Can you work these out from the model? Positions are in its coordinate system, mm. A direction names the side the tool comes from. Give positions to 0.01 mm unless a question says otherwise; leave off trailing zeros. Loops run counter-clockwise (first coordinate to the right, second up) from the corner with the lowest first, then second, coordinate; pieces in that order, holes last.
Autodesk Fusion 360 part; units mm, degrees
sketch "Sketch1" plane through (0, 0, 0) normal (0, 1, 0) x (1, 0, 0)
  line L0 (-22.3654, 14.0021) -> (11.8346, 14.0021)
  line L1 (11.8346, 14.0021) -> (11.8346, -7.1979)
  line L2 (11.8346, -7.1979) -> (-22.3654, -7.1979)
  line L3 (-22.3654, -7.1979) -> (-22.3654, 14.0021)
  line L4 (-19.5354, 11.0221) -> (-16.9954, 11.0221)
  line L5 (-16.9954, 11.0221) -> (-16.9954, -4.2179)
  line L6 (-16.9954, -4.2179) -> (-19.5354, -4.2179)
  line L7 (-19.5354, -4.2179) -> (-19.5354, 11.0221)
  line L8 (6.4646, 8.4821) -> (9.0046, 8.4821)
  line L9 (9.0046, 8.4821) -> (9.0046, -1.6779)
  line L10 (9.0046, -1.6779) -> (6.4646, -1.6779)
  line L11 (6.4646, -1.6779) -> (6.4646, 8.4821)
  line L12 (11.8346, 3.4021) -> (-22.3654, 3.4021) construction
  line L13 (-16.2654, 14.0021) -> (5.7346, 14.0021)
  line L14 (5.7346, 14.0021) -> (5.7346, -7.1979)
  line L15 (5.7346, -7.1979) -> (-16.2654, -7.1979)
  line L16 (-16.2654, -7.1979) -> (-16.2654, 14.0021)
  line L17 (-18.2654, -4.2179) -> (-18.2654, 11.0221) construction
  line L18 (7.7346, -1.6779) -> (7.7346, 8.4821) construction
  circle A0 centre (7.7346, 11.0021) radius 1.5
  circle A1 centre (7.7346, -4.1979) radius 1.5
  line L19 (7.7346, -4.1979) -> (7.7346, 11.0021) construction
  point P0 (-16.9954, 3.4021)
  point P1 (-19.5354, 3.4021)
  point P2 (6.4646, 3.4021)
  point P3 (9.0046, 3.4021)
  dimension "d1" = 34.2
  dimension "d2" = 21.2
  dimension "d3" = 15.24
  dimension "d4" = 2.54
  dimension "d5" = 10.16
  dimension "d6" = 2.54
  dimension "d7" = 22
  dimension "d8" = 4.1
  dimension "d9" = 4.1
  dimension "d16" = 3
  dimension "d17" = 3
  dimension "d18" = 15.2
extrude "Extrude1" add sketch "Sketch1" against normal blind 1.7 contours L0 L2 L3 L16 | L0 L2 L13 L14 L15 L16 | L0 L1 L2 L14 | L4 L5 L6 L7 | L8 L9 L10 L11 | A0 | A1
extrude "Extrude2" add sketch "Sketch1" along normal blind 2.2 contours L0 L2 L13 L14 L15 L16
extrude "Extrude3" add sketch "Sketch1" along normal blind 4.5 contours L4 L5 L6 L7 | L8 L9 L10 L11
extrude "Extrude4" cut sketch "Sketch1" against normal blind 5 contours A0 | A1
(1) Suppose I cut it at A-A on y = 1.25. List the corners of the cut face in (x, z) for me.
Returned:
outline: (-19.54, -11.02) - (-17, -11.02) - (-17, 4.22) - (-19.54, 4.22) - close; (-16.27, -14) - (5.73, -14) - (5.73, 7.2) - (-16.27, 7.2) - close; (6.46, -8.48) - (9, -8.48) - (9, 1.68) - (6.46, 1.68) - close
(2) Thinking about a two-plate mould opening in X: for faces 5 (the flat face through (-6, -1.7, -4)), 6 (the flat face through (5.735, 1, -4)), 7 (the flat face through (-22.365, -1, -3)), which applies, pulls with the +X half, pulls with the -X half, needs draft (parallel to the pull), parting line crosses it, or undercut?
Returned:
face 5: needs draft
face 6: undercut
face 7: pulls with the -X half
(3) Suppose I cut it at C-C on z = 3.75. List the corners of the cut face in (x, y) for me.
Returned:
outline: (-22.37, -1.7) - (6.3, -1.7) - (6.3, 0) - (5.73, 0) - (5.73, 2.2) - (-16.27, 2.2) - (-16.27, 0) - (-17, 0) - (-17, 4.5) - (-19.54, 4.5) - (-19.54, 0) - (-22.37, 0) - close; (9.17, -1.7) - (11.83, -1.7) - (11.83, 0) - (9.17, 0) - close
(4) Suppose I cut it at D-D on y = -0.75. List the corners of the cut face in (x, z) for me.
Returned:
outline: (-22.37, -14) - (11.83, -14) - (11.83, 7.2) - (-22.37, 7.2) - close; hole circle Ø3 at (7.73, -11); hole circle Ø3 at (7.73, 4.2)
(5) Which directions (+Z, -Z, +X, -X, +Y, -Y) give clear straight access to the entire face, cutting with the end or side of a thin tool? Please do faces 1 (the flat face through (-19.535, 2, -3)), 2 (the flat face through (-18, 2, 4.218)), 3 (the flat face through (6.465, 2, -3)), 4 (the flat face through (8, 2, -8.482)).
Returned:
face 1: +Z, -Z, -X, +Y
face 2: +Z, -X, +Y
face 3: +Z, -Z, +Y
face 4: -Z, +X, +Y
(6) Suppose I cut it at B-B on z = -6. List the corners of the cut face in (x, y) for me.
Returned:
outline: (-22.37, -1.7) - (11.83, -1.7) - (11.83, 0) - (9, 0) - (9, 4.5) - (6.46, 4.5) - (6.46, 0) - (5.73, 0) - (5.73, 2.2) - (-16.27, 2.2) - (-16.27, 0) - (-17, 0) - (-17, 4.5) - (-19.54, 4.5) - (-19.54, 0) - (-22.37, 0) - close
(7) Please list where these lines run through material, in increasing order: probe 1 along X at (y, z) = (0.25, 1.25); probe 2 along X at (y, z) = (0.25, 2.25); probe 3 along Y at (x, z) = (3, -6).
Returned:
probe 1: x = -19.54 to -17, -16.27 to 5.73, 6.46 to 9
probe 2: x = -19.54 to -17, -16.27 to 5.73
probe 3: y = -1.7 to 2.2
(8) Will these pins go through, and if not, where does the flat tip stop? P1, Ø1.3, axis at x = -18, y = 3.5, coming from the -Z side; P2, Ø1, axis at x = -1, z = -7, coming from the +Y side; P3, Ø1.3, axis at x = -17.5, y = 3, coming from the +Z side; P4, Ø1.8, axis at x = 7.73, z = 4.2, coming from the -Y side.
Returned:
P1: stops at z = -11.02
P2: stops at y = 2.2
P3: stops at z = 4.22
P4: passes through
